Check sheet for the modelled part. Datum: model origin and axes. Units: mm. A direction names the side the tool comes from. Give positions to 0.01 mm unless a question says otherwise; leave off trailing zeros. Loops run counter-clockwise (first coordinate to the right, second up) from the corner with the lowest first, then second, coordinate; pieces in that order, holes last. Notation, with made-up numbers: (35, 88) - (65, 88) arc R28 cw to (65, 112) - close; hole circle Ø7 at (27, 73.5). An arc over 180 degrees is marked (long way). Answer in a Markdown table with one row per item. Add a question column.
(1) Set-up check for faces 1 (the face through (17, 4, -2.4)), 2 (the face through (14.414, 8.915, -3.58)), 3 (the face through (13, 5, -10)), 4 (the face through (2.54, 6.22, -4.73)): record each of +Z, -Z, +X, -X, +Y, -Y from which the full face is reachable in a straight line by a thin tool's end or side.
(2) Sectioned sample at D-D on x = 3.25. Enter the section's corners in (y, z).
(3) Sectioned sample at C-C on x = 12. Enter the section's corners in (y, z).
(4) Go/stop test with flat-tipped pins: P1, Ø0.7, axis at x = 6, y = 6, coming from the +Z side; P2, Ø2, axis at x = 12, z = -5, coming from the +Y side. Record where each tip stops, or that it passes through.
(5) Sectioned sample at B-B on z = -6. Enter the section's corners in (x, y).
(6) Thickness scan on L1, parallel to X at y = 7.5, z = -2.75; L2, parallel to Y at x = 1.6, z = -5; L3, parallel to X at y = 5.5, z = -7. Record the ranges inside material, lowest first.
(7) Sectioned sample at A-A on y = 5. Enter the section's corners in (x, z).
(8) Draft check along Y on faces 5 (the face through (13.4, 7.8, -5)), 6 (the face through (6, 2.2, -4)), 7 (the face through (12, 9, -7.8)). Enter one of: released by +Y, released by -Y, zero draft, split by the parting line, or undercut.
from build123d import *

# Parameters (mm, degrees)
SKETCH1_W           = 74.5
SKETCH1_H           = 10
BOSS_EXTRUDE1_DEPTH = 10
SKETCH2_R           = 1.25
CUT_EXTRUDE1_DEPTH  = 10
SKETCH3_R           = 1.25
CUT_EXTRUDE2_DEPTH  = 10
SKETCH4_R           = 1.25
CUT_EXTRUDE3_DEPTH  = 5
CUT_EXTRUDE4_START  = -5
SKETCH5_R           = 1.25
CUT_EXTRUDE4_DEPTH  = 5
CUT_EXTRUDE5_DEPTH  = 2.2
CUT_EXTRUDE6_DEPTH  = 2.2
CUT_EXTRUDE8_DEPTH  = 2.2
SKETCH11_W          = 2.3
SKETCH11_H          = 5.6
CUT_EXTRUDE9_DEPTH  = 7.3
SKETCH12_W          = 92.79599186
SKETCH12_H          = 35.188487641
CUT_EXTRUDE10_DEPTH = 14
CUT_EXTRUDE11_DEPTH = 2.4
FILLET1_R           = 2
FILLET2_R           = 2


with BuildPart() as part:
    # Sketch1 → Boss-Extrude1 (new body)
    with BuildSketch(Plane(origin=(0, 0, 0), x_dir=(1, 0, 0), z_dir=(0, 1, 0))):
        with Locations((37.25, 5)):
            Rectangle(SKETCH1_W, SKETCH1_H)
    extrude(amount=BOSS_EXTRUDE1_DEPTH)

    # Sketch2 → Cut-Extrude1 (cut)
    with BuildSketch(Plane(origin=(0, 10, 0), x_dir=(1, 0, 0), z_dir=(0, 1, 0))):
        with Locations(Location((12, 5, 0), (0, 0, 270))):
            Circle(SKETCH2_R)
        with Locations(Location((62.5, 5, 0), (0, 0, 270))):
            Circle(SKETCH2_R)
    extrude(amount=-CUT_EXTRUDE1_DEPTH, mode=Mode.SUBTRACT)

    # Sketch3 → Cut-Extrude2 (cut)
    with BuildSketch(Plane(origin=(0, 0, -10), x_dir=(-1, 0, 0), z_dir=(0, 0, -1))):
        with Locations((-56.5, 5)):
            Circle(SKETCH3_R)
        with Locations((-18, 5)):
            Circle(SKETCH3_R)
    extrude(amount=-CUT_EXTRUDE2_DEPTH, mode=Mode.SUBTRACT)

    # Sketch4 → Cut-Extrude3 (cut)
    with BuildSketch(Plane(origin=(74.5, 0, 0), x_dir=(0, 0, -1), z_dir=(1, 0, 0))):
        with Locations((5, 5)):
            Circle(SKETCH4_R)
    extrude(amount=-CUT_EXTRUDE3_DEPTH, mode=Mode.SUBTRACT)

    # Sketch5 → Cut-Extrude4 (cut)
    with BuildSketch(Plane.ZY.offset(CUT_EXTRUDE4_START)):
        with Locations(Location((-5, 5, 0), (0, 0, 180))):
            Circle(SKETCH5_R)
    extrude(amount=CUT_EXTRUDE4_DEPTH, mode=Mode.SUBTRACT)

    # Sketch6 → Cut-Extrude5 (cut)
    with BuildSketch(Plane(origin=(0, 10, 0), x_dir=(1, 0, 0), z_dir=(0, 1, 0))):
        Polygon((13.616580754, 2.2), (15.233161507, 5), (13.616580754, 7.8), (10.383419246, 7.8), (8.766838493, 5), (10.383419246, 2.2), align=None)
    extrude(amount=-CUT_EXTRUDE5_DEPTH, mode=Mode.SUBTRACT)

    # Sketch7 → Cut-Extrude6 (cut)
    with BuildSketch(Plane(origin=(0, 10, 0), x_dir=(1, 0, 0), z_dir=(0, 1, 0))):
        Polygon((60.883419246, 7.8), (59.266838493, 5), (60.883419246, 2.2), (64.116580754, 2.2), (65.733161507, 5), (64.116580754, 7.8), align=None)
    extrude(amount=-CUT_EXTRUDE6_DEPTH, mode=Mode.SUBTRACT)

    # Sketch9 → Cut-Extrude8 (cut)
    with BuildSketch(Plane.XY):
        Polygon((58.116580754, 7.8), (54.883419246, 7.8), (53.266838493, 5), (54.883419246, 2.2), (58.116580754, 2.2), (59.733161507, 5), align=None)
    extrude(amount=-CUT_EXTRUDE8_DEPTH, mode=Mode.SUBTRACT)

    # Sketch11 → Cut-Extrude9 (cut)
    with BuildSketch(Plane.XY):
        with Locations((6.15, 5)):
            Rectangle(SKETCH11_W, SKETCH11_H)
        with Locations((68.35, 5)):
            Rectangle(SKETCH11_W, SKETCH11_H)
    extrude(amount=-CUT_EXTRUDE9_DEPTH, mode=Mode.SUBTRACT)

    # Sketch12 → Cut-Extrude10 (cut)
    with BuildSketch(Plane.XY):
        with Locations((72.539564665, 12.110455679)):
            Rectangle(SKETCH12_W, SKETCH12_H)
    extrude(amount=-CUT_EXTRUDE10_DEPTH, mode=Mode.SUBTRACT)

    # Sketch13 → Cut-Extrude11 (cut)
    with BuildSketch(Plane.XY):
        Polygon((20.8, 6.616580754), (18, 8.233161507), (15.2, 6.616580754), (15.2, 3.383419246), (18, 1.766838493), (20.8, 3.383419246), align=None)
    extrude(amount=-CUT_EXTRUDE11_DEPTH, mode=Mode.SUBTRACT)

    # Fillet1
    fillet1_edges = [part.edges().sort_by_distance(p)[0] for p in [
        (26.141568735, 5, 0),
    ]]
    fillet(fillet1_edges, radius=FILLET1_R)

    # Fillet2
    # the kernel refuses this fillet: 2 mm, written as the material it takes off along each edge
    with BuildSketch(Plane(origin=(26.141568735, 10, -15), x_dir=(-1, 0, 0), z_dir=(0, 0, 1))) as fillet2_piece_1:
        with BuildLine():
            CenterArc((FILLET2_R, FILLET2_R), FILLET2_R, 180, 90)
            Line((0, FILLET2_R), (0, 0))
            Line((0, 0), (FILLET2_R, 0))
        make_face()
    extrude(amount=13, mode=Mode.SUBTRACT)
    with BuildSketch(Plane(origin=(24.141568735, 10, -2), x_dir=(0, 0, 1), z_dir=(-1, 0, 0))) as fillet2_piece_2:
        with BuildLine():
            CenterArc((2 - FILLET2_R, -FILLET2_R), FILLET2_R, 0, 90)
            Line((2 - FILLET2_R, 0), (2, 0))
            Line((2, 0), (2, -FILLET2_R))
        make_face()
    revolve(axis=Axis((24.141568735, 10, -2), (0, 1, 0)), revolution_arc=90, mode=Mode.SUBTRACT)
    with BuildSketch(Plane(origin=(-5, 10, 0), x_dir=(0, -1, 0), z_dir=(1, 0, 0))) as fillet2_piece_3:
        with BuildLine():
            CenterArc((FILLET2_R, FILLET2_R), FILLET2_R, 180, 90)
            Line((0, FILLET2_R), (0, 0))
            Line((0, 0), (FILLET2_R, 0))
        make_face()
    extrude(amount=29.141568735, mode=Mode.SUBTRACT)


solid = part.part
Reply:
| question | item | result |
|---|---|---|
| 1 | face 1 | +Z |
| 1 | face 2 | +Y |
| 1 | face 3 | -Z, +X, -X, +Y, -Y |
| 1 | face 4 | -X |
| 2 | outline | (0, -10) - (10, -10) - (10, -2) arc R2 ccw to (8, 0) - (0, 0) - close; hole circle Ø2.5 at (5, -5) |
| 3 | outline | (0, -10) - (10, -10) - (10, -7.8) - (7.8, -7.8) - (7.8, -6.25) - (0, -6.25) - close; (0, -3.75) - (7.8, -3.75) - (7.8, -2.2) - (10, -2.2) - (10, -2) arc R2 ccw to (8, 0) - (0, 0) - close |
| 4 | P1 | z = -7.3 |
| 4 | P2 | through |
| 5 | outline | (0, 0) - (11.25, 0) - (11.25, 7.8) - (9.34, 7.8) - (9.34, 10) - (0, 10) - (0, 5.75) - (5, 5.75) - (5, 7.8) - (7.3, 7.8) - (7.3, 2.2) - (5, 2.2) - (5, 4.25) - (0, 4.25) - close; (12.75, 0) - (26.14, 0) - (26.14, 8) arc R2 ccw to (24.14, 10) - (14.66, 10) - (14.66, 7.8) - (12.75, 7.8) - close; hole circle Ø2.5 at (18, 5) |
| 6 | L1 | 0 to 5, 7.3 to 26.14 |
| 6 | L2 | 0 to 3.75, 6.25 to 10 |
| 6 | L3 | 0 to 5, 7.3 to 16.85, 19.15 to 26.14 |
| 7 | outline | (0, -10) - (16.75, -10) - (16.75, -2.4) - (15.2, -2.4) - (15.2, 0) - (7.3, 0) - (7.3, -7.3) - (5, -7.3) - (5, -6.25) - (0, -6.25) - close; (0, -3.75) - (5, -3.75) - (5, 0) - (0, 0) - close; (19.25, -10) - (26.14, -10) - (26.14, -2) arc R2 ccw to (24.14, 0) - (20.8, 0) - (20.8, -2.4) - (19.25, -2.4) - close; hole circle Ø2.5 at (12, -5) |
| 8 | face 5 | released by +Y |
| 8 | face 6 | undercut |
| 8 | face 7 | zero draft |
